from build123d import *

# Parameters (mm, degrees)
SKETCH1_R           = 270
SKETCH1_R_2         = 240
BOSS_EXTRUDE1_DEPTH = 50
FILLET1_R           = 25
BOSS_EXTRUDE2_DEPTH = 50
SKETCH3_R           = 50
BOSS_EXTRUDE3_DEPTH = 50
SKETCH4_R           = 27
CUT_EXTRUDE1_DEPTH  = 50
SKETCH5_R           = 27
CUT_EXTRUDE2_DEPTH  = 50
FILLET2_R           = 120
FILLET3_R           = 120
FILLET4_R           = 120
FILLET5_R           = 120
FILLET6_R           = 120
FILLET7_R           = 120
FILLET8_R           = 70
FILLET9_R           = 70
FILLET10_R          = 70
FILLET11_R          = 70
FILLET12_R          = 70
FILLET13_R          = 70
FILLET14_R          = 70
FILLET15_R          = 70
FILLET16_R          = 70
FILLET17_R          = 70
FILLET18_R          = 70
FILLET19_R          = 70
FILLET20_R          = 20
FILLET21_R          = 20
FILLET22_R          = 20
FILLET23_R          = 20
FILLET24_R          = 20
FILLET25_R          = 20
FILLET26_R          = 10
FILLET27_R          = 10
FILLET28_R          = 10


with BuildPart() as part:
    # Sketch1 → Boss-Extrude1 (new body)
    with BuildSketch(Plane(origin=(0, 0, 0), x_dir=(0, 0, -1), z_dir=(1, 0, 0))):
        Circle(SKETCH1_R)
        Circle(SKETCH1_R_2, mode=Mode.SUBTRACT)
    extrude(amount=BOSS_EXTRUDE1_DEPTH)

    # Fillet1
    fillet1_edges = [part.edges().sort_by_distance(p)[0] for p in [
        (0, 0, 270),
        (50, 0, 270),
    ]]
    fillet(fillet1_edges, radius=FILLET1_R - 0.0001)  # a hair under: the kernel refuses the full size

    # Sketch2 → Boss-Extrude2 (add)
    with BuildSketch(Plane(origin=(0, 0, 0), x_dir=(0, 0, -1), z_dir=(1, 0, 0))):
        with BuildLine():
            Line((10.910154565, 6.298980675), (36.524952377, 183.573393863))
            Line((36.524952377, 183.573393863), (10, 239.791576166))
            ThreePointArc((10, 239.791576166), (0, 240), (-10, 239.791576166))
            Line((-10, 239.791576166), (-36.524952377, 183.573393863))
            Line((-36.524952377, 183.573393863), (-10.910154565, 6.298980675))
            Line((-10.910154565, 6.298980675), (-177.241698733, -60.155160301))
            Line((-177.241698733, -60.155160301), (-212.665596573, -111.235534045))
            ThreePointArc((-212.665596573, -111.235534045), (-207.846096908, -120), (-202.665596573, -128.556042121))
            Line((-202.665596573, -128.556042121), (-140.716746356, -123.418233562))
            Line((-140.716746356, -123.418233562), (0, -12.59796135))
            Line((0, -12.59796135), (140.716746356, -123.418233562))
            Line((140.716746356, -123.418233562), (202.665596573, -128.556042121))
            ThreePointArc((202.665596573, -128.556042121), (207.846096908, -120), (212.665596573, -111.235534045))
            Line((212.665596573, -111.235534045), (177.241698733, -60.155160301))
            Line((177.241698733, -60.155160301), (10.910154565, 6.298980675))
        make_face()
    extrude(amount=BOSS_EXTRUDE2_DEPTH)

    # Sketch3 → Boss-Extrude3 (add)
    with BuildSketch(Plane(origin=(50, 0, 0), x_dir=(0, 0, -1), z_dir=(1, 0, 0))):
        Circle(SKETCH3_R)
    extrude(amount=-BOSS_EXTRUDE3_DEPTH)

    # Sketch4 → Cut-Extrude1 (cut)
    with BuildSketch(Plane(origin=(50, 0, 0), x_dir=(0, 0, -1), z_dir=(1, 0, 0))):
        Circle(SKETCH4_R)
    extrude(amount=-CUT_EXTRUDE1_DEPTH, mode=Mode.SUBTRACT)

    # Sketch5 → Cut-Extrude2 (cut)
    with BuildSketch(Plane(origin=(50, 0, 0), x_dir=(0, 0, -1), z_dir=(1, 0, 0))):
        Circle(SKETCH5_R)
        with BuildLine():
            Line((-6.907151282, 48.521613039), (-26.197593694, 182.026545767))
            Line((-26.197593694, 182.026545767), (-0.956115014, 235.524475937))
            Line((-0.956115014, 235.524475937), (0, 237.550909289))
            Line((0, 237.550909289), (0.956115014, 235.524475937))
            Line((0.956115014, 235.524475937), (26.197593694, 182.026545767))
            Line((26.197593694, 182.026545767), (6.907151282, 48.521613039))
            ThreePointArc((6.907151282, 48.521613039), (0, 49.010770967), (-6.907151282, 48.521613039))
        make_face()
        with BuildLine():
            Line((45.474525166, -18.279038041), (170.738409645, -68.325491226))
            Line((170.738409645, -68.325491226), (204.448236882, -116.934218077))
            Line((204.448236882, -116.934218077), (205.725122137, -118.775454645))
            Line((205.725122137, -118.775454645), (203.492121867, -118.59025786))
            Line((203.492121867, -118.59025786), (144.54081595, -113.701054541))
            Line((144.54081595, -113.701054541), (38.567373883, -30.242574998))
            ThreePointArc((38.567373883, -30.242574998), (42.444572716, -24.505385483), (45.474525166, -18.279038041))
        make_face()
        with BuildLine():
            Line((-38.567373883, -30.242574998), (-144.54081595, -113.701054541))
            Line((-144.54081595, -113.701054541), (-203.492121867, -118.59025786))
            Line((-203.492121867, -118.59025786), (-205.725122137, -118.775454645))
            Line((-205.725122137, -118.775454645), (-204.448236882, -116.934218077))
            Line((-204.448236882, -116.934218077), (-170.738409645, -68.325491226))
            Line((-170.738409645, -68.325491226), (-45.474525166, -18.279038041))
            ThreePointArc((-45.474525166, -18.279038041), (-42.444572716, -24.505385483), (-38.567373883, -30.242574998))
        make_face()
    extrude(amount=-CUT_EXTRUDE2_DEPTH, mode=Mode.SUBTRACT)

    # Fillet2
    fillet2_edges = [part.edges().sort_by_distance(p)[0] for p in [
        (25, -38.098779813, -32.380286854),
    ]]
    fillet(fillet2_edges, radius=FILLET2_R)

    # Fillet3
    fillet3_edges = [part.edges().sort_by_distance(p)[0] for p in [
        (25, -8.992761091, -49.184654598),
    ]]
    fillet(fillet3_edges, radius=FILLET3_R)

    # Fillet4
    fillet4_edges = [part.edges().sort_by_distance(p)[0] for p in [
        (25, -38.098779813, 32.380286854),
    ]]
    fillet(fillet4_edges, radius=FILLET4_R)

    # Fillet5
    fillet5_edges = [part.edges().sort_by_distance(p)[0] for p in [
        (25, -8.992761091, 49.184654598),
    ]]
    fillet(fillet5_edges, radius=FILLET5_R)

    # Fillet6
    fillet6_edges = [part.edges().sort_by_distance(p)[0] for p in [
        (25, 47.091540904, 16.804367744),
    ]]
    fillet(fillet6_edges, radius=FILLET6_R)

    # Fillet7
    fillet7_edges = [part.edges().sort_by_distance(p)[0] for p in [
        (25, 47.091540904, -16.804367744),
    ]]
    fillet(fillet7_edges, radius=FILLET7_R)

    # Fillet8
    fillet8_edges = [part.edges().sort_by_distance(p)[0] for p in [
        (25, -123.418233562, -140.716746356),
    ]]
    fillet(fillet8_edges, radius=FILLET8_R)

    # Fillet9
    fillet9_edges = [part.edges().sort_by_distance(p)[0] for p in [
        (25, -60.155160301, -177.241698733),
    ]]
    fillet(fillet9_edges, radius=FILLET9_R)

    # Fillet10
    fillet10_edges = [part.edges().sort_by_distance(p)[0] for p in [
        (25, -123.418233562, 140.716746356),
    ]]
    fillet(fillet10_edges, radius=FILLET10_R)

    # Fillet11
    fillet11_edges = [part.edges().sort_by_distance(p)[0] for p in [
        (25, -60.155160301, 177.241698733),
    ]]
    fillet(fillet11_edges, radius=FILLET11_R)

    # Fillet12
    fillet12_edges = [part.edges().sort_by_distance(p)[0] for p in [
        (25, 183.573393863, 36.524952377),
    ]]
    fillet(fillet12_edges, radius=FILLET12_R)

    # Fillet13
    fillet13_edges = [part.edges().sort_by_distance(p)[0] for p in [
        (25, 183.573393863, -36.524952377),
    ]]
    fillet(fillet13_edges, radius=FILLET13_R)

    # Fillet14
    fillet14_edges = [part.edges().sort_by_distance(p)[0] for p in [
        (25, -113.701054541, -144.54081595),
    ]]
    fillet(fillet14_edges, radius=FILLET14_R)

    # Fillet15
    fillet15_edges = [part.edges().sort_by_distance(p)[0] for p in [
        (25, -68.325491226, -170.738409645),
    ]]
    fillet(fillet15_edges, radius=FILLET15_R)

    # Fillet16
    fillet16_edges = [part.edges().sort_by_distance(p)[0] for p in [
        (25, -68.325491226, 170.738409645),
    ]]
    fillet(fillet16_edges, radius=FILLET16_R)

    # Fillet17
    fillet17_edges = [part.edges().sort_by_distance(p)[0] for p in [
        (25, -113.701054541, 144.54081595),
    ]]
    fillet(fillet17_edges, radius=FILLET17_R)

    # Fillet18
    fillet18_edges = [part.edges().sort_by_distance(p)[0] for p in [
        (25, 182.026545767, -26.197593694),
    ]]
    fillet(fillet18_edges, radius=FILLET18_R)

    # Fillet19
    fillet19_edges = [part.edges().sort_by_distance(p)[0] for p in [
        (25, 182.026545767, 26.197593694),
    ]]
    fillet(fillet19_edges, radius=FILLET19_R)

    # Fillet20
    fillet20_edges = [part.edges().sort_by_distance(p)[0] for p in [
        (25, 239.791576166, -10),
    ]]
    fillet(fillet20_edges, radius=FILLET20_R)

    # Fillet21
    fillet21_edges = [part.edges().sort_by_distance(p)[0] for p in [
        (25, 239.791576166, 10),
    ]]
    fillet(fillet21_edges, radius=FILLET21_R)

    # Fillet22
    fillet22_edges = [part.edges().sort_by_distance(p)[0] for p in [
        (25, -111.235534045, -212.665596573),
    ]]
    fillet(fillet22_edges, radius=FILLET22_R)

    # Fillet23
    fillet23_edges = [part.edges().sort_by_distance(p)[0] for p in [
        (25, -128.556042121, -202.665596573),
    ]]
    fillet(fillet23_edges, radius=FILLET23_R)

    # Fillet24
    fillet24_edges = [part.edges().sort_by_distance(p)[0] for p in [
        (25, -128.556042121, 202.665596573),
    ]]
    fillet(fillet24_edges, radius=FILLET24_R)

    # Fillet25
    fillet25_edges = [part.edges().sort_by_distance(p)[0] for p in [
        (25, -111.235534045, 212.665596573),
    ]]
    fillet(fillet25_edges, radius=FILLET25_R)

    # Fillet26
    fillet26_edges = [part.edges().sort_by_distance(p)[0] for p in [
        (25, -118.775454645, -205.725122137),
    ]]
    fillet(fillet26_edges, radius=FILLET26_R)

    # Fillet27
    fillet27_edges = [part.edges().sort_by_distance(p)[0] for p in [
        (25, -118.775454645, 205.725122137),
    ]]
    fillet(fillet27_edges, radius=FILLET27_R)

    # Fillet28
    fillet28_edges = [part.edges().sort_by_distance(p)[0] for p in [
        (25, 237.550909289, 0),
    ]]
    fillet(fillet28_edges, radius=FILLET28_R)


solid = part.part
Read the model definition and answer for the solid it produces. Units are mm, in the model's axes. Coordinates: 2 decimals unless noted, no trailing zeros. Use a Markdown table: item, result.
Q1. Determine the mould class of faces 1 (the face through (25.35, -62.401, 175.088)), 2 (the face through (25.35, -26.36, 5.85)) for opening direction Z: released by +Z, released by -Z, zero draft, split by the parting line, or undercut.
Answer block:
| item | result |
|---|---|
| face 1 | undercut |
| face 2 | undercut |
Q2. The part is cut by section A-A, the plane y = 0. Give the number of separate pieces and of enclosed holes in the cut face, then the cut area to 3 significant figures.
Answer block:
| item | result |
|---|---|
| separate pieces | 4 |
| enclosed holes | 0 |
| area | 5,820 mm2 |
Q3. Each of these flat-tipped pins is pushed along its axis until it touches: pin 1 Ø10 at (x, z) = (8.5, 112) entering from +Y; pin 2 Ø6 at (x, y) = (19, -88.5) entering from +Z; pin 3 Ø5 at (x, z) = (44, 169) entering from +Y. Where does it stop, or does it pass through?
Answer block:
| item | result |
|---|---|
| pin 1 | stops at y = 243.36 |
| pin 2 | stops at z = 255.54 |
| pin 3 | stops at y = 203.19 |
Q4. Straight lines are drawn through the part: L1, parallel to Z at x = 30.5, y = -61.5; L2, parallel to Y at x = 32, z = 128; L3, parallel to Y at x = 34, z = 78.5. For each, find the intervals that lie inside material, in ascending order. Write a range as [from, to].
Answer block:
| item | result |
|---|---|
| L1 | z = [-262.27, -231.99], [-173.92, -153.53], [-78.26, -57.26], [57.26, 78.26], [153.53, 173.92], [231.99, 262.27] |
| L2 | y = [-236.59, -203.02], [-113.2, -100.67], [-51.25, -40.48], [203.02, 236.59] |
| L3 | y = [-256.58, -226.8], [-74.44, -61.69], [-31.47, -16.41], [226.8, 256.58] |
